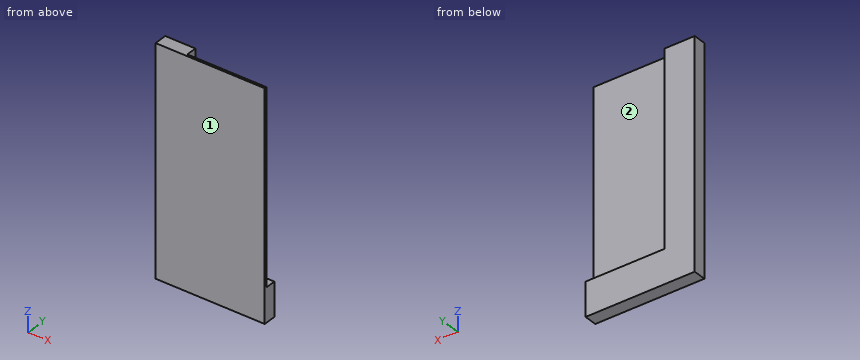
Autodesk Inventor part; units mm, degrees
ref_plane "YZ Plane" through (0, 0, 0) normal (1, 0, 0) x (0, 1, 0)
ref_plane "XZ Plane" through (0, 0, 0) normal (0, 1, 0) x (-1, 0, 0)
ref_plane "XY Plane" through (0, 0, 0) normal (0, 0, 1) x (1, 0, 0)
sketch "Sketch1" plane through (0, 0, 0) normal (0, 1, 0) x (-1, 0, 0)
  line L0 (0, 0) -> (184.15, 0)
  line L1 (184.15, 0) -> (184.15, 381)
  line L2 (184.15, 381) -> (0, 381)
  line L3 (0, 381) -> (0, 0)
  dimension "d0" = 184.15
  dimension "d1" = 381
extrude "Extrusion1" add sketch "Sketch1" along normal blind 21.6408
sketch "Sketch2" plane through (0, 21.6408, 0) normal (0, 1, 0) x (1, 0, 0)
  line L0 (0, -381) -> (-133.35, -381)
  line L1 (-133.35, -381) -> (-133.35, -57.15)
  line L2 (-133.35, -57.15) -> (0, -57.15)
  line L3 (0, -57.15) -> (0, -381)
  line L4 (0, -381) -> (0, 0)
  line L5 (-184.15, -381) -> (0, -381)
  dimension "d4" = 133.35
  dimension "d5" = 323.85
  dimension "d6" = 0
  dimension "d7" = 0
extrude "Extrusion2" cut sketch "Sketch2" against normal blind 18.0086
properties part number "Case stock 1"
Model file for the job. Use its own axes, mm. Face numbers are marked on the shaded views. A direction names the side the tool comes from. Give positions to 0.01 mm unless a question says otherwise; leave off trailing zeros. Write each loop counter-clockwise with the first axis right and the second up, starting at its lowest first coordinate (ties: lowest second). Pieces come first, ordered by that corner, then holes. Notation, with made-up numbers: M -29.5,59 L -22.5,59 A27 cw -22.5,97 Z; hole C 2,73.5 d7. An arc over 180 degrees is marked long. One line per item, written item: value. Start each with the question number.
Q1. Saw through at B-B, the plane x = -90. Write the cut outline in (y, z).
Q2. 3-axis set-ups, long thin cutter, end or side, ignore diameter. For the marked faces 1 and 2: which of +Z, -Z, +X, -X, +Y, -Y reach the whole face in a straight line?
Q3. Saw through at A-A, the plane y = 8.75. Write the cut outline in (x, z).
Q4. Probe probe 1 along X at (y, z) = (15.25, 227); probe 2 along Z at (x, y) = (-28.5, 4.25); probe 3 along Y at (x, z) = (-124, 105). List the from-to ranges inside material, lowest first. Write a range as [from, to].
Output values:
1. outline: M 0,0 L 21.64,0 L 21.64,57.15 L 3.63,57.15 L 3.63,381 L 0,381 Z
2. face 1: +Z, -Z, +X, -X, -Y
2. face 2: +Z, +X, +Y
3. outline: M -184.15,0 L 0,0 L 0,57.15 L -133.35,57.15 L -133.35,381 L -184.15,381 Z
4. probe 1: x = [-184.15, -133.35]
4. probe 2: z = [0, 57.15]
4. probe 3: y = [0, 3.63]
